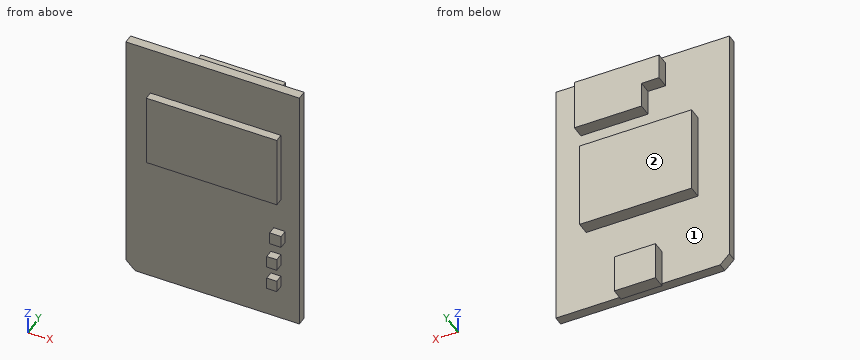
from build123d import *

# Parameters (mm, degrees)
BOSS_EXTRUDE1_DEPTH = 1.6
SKETCH3_W           = 19.355079094
SKETCH3_H           = 15.609116434
BOSS_EXTRUDE2_DEPTH = 2.2
SKETCH4_W           = 7.104895368
SKETCH4_H           = 6.377418
SKETCH4_H_2         = 0.4
BOSS_EXTRUDE4_DEPTH = 2.2
SKETCH5_W           = 22.566472962
SKETCH5_H           = 12.815854083
BOSS_EXTRUDE5_DEPTH = 1.4
SKETCH6_W           = 1.734301273
SKETCH6_H           = 2.066889472
SKETCH6_H_2         = 2.110641646
SKETCH6_W_2         = 1.994894676
SKETCH6_H_3         = 2.153908206
BOSS_EXTRUDE6_DEPTH = 1.4
SKETCH7_W           = 11.606028653
SKETCH7_H           = 9.032244077
SKETCH7_W_2         = 3.035472579
SKETCH7_H_2         = 4.516122038
BOSS_EXTRUDE7_DEPTH = 2.2


with BuildPart() as part:
    # Sketch2 → Boss-Extrude1 (new body)
    with BuildSketch(Plane(origin=(0, 0, 0), x_dir=(1, 0, 0), z_dir=(0, 1, 0))):
        Polygon((1.6, 45), (0, 43.4), (0, 0), (30, 0), (30, 45), align=None)
    extrude(amount=BOSS_EXTRUDE1_DEPTH)

    # Sketch3 → Boss-Extrude2 (add)
    with BuildSketch(Plane(origin=(0, 1.6, 0), x_dir=(1, 0, 0), z_dir=(0, 1, 0))):
        with Locations((15.091884819, 22.082133677)):
            Rectangle(SKETCH3_W, SKETCH3_H)
    extrude(amount=BOSS_EXTRUDE2_DEPTH)

    # Sketch4 → Boss-Extrude4 (add)
    with BuildSketch(Plane(origin=(0, 1.6, 0), x_dir=(1, 0, 0), z_dir=(0, 1, 0))):
        with Locations((15.215017688, 41.811291)):
            Rectangle(SKETCH4_W, SKETCH4_H)
        with Locations((15.215017688, 45.2)):
            Rectangle(SKETCH4_W, SKETCH4_H_2)
    extrude(amount=BOSS_EXTRUDE4_DEPTH)

    # Sketch5 → Boss-Extrude5 (add)
    with BuildSketch(Plane(origin=(0, 0, 0), x_dir=(-1, 0, 0), z_dir=(0, -1, 0))):
        with Locations((-15.528488828, 15.010487551)):
            Rectangle(SKETCH5_W, SKETCH5_H)
    extrude(amount=BOSS_EXTRUDE5_DEPTH)

    # Sketch6 → Boss-Extrude6 (add)
    with BuildSketch(Plane(origin=(0, 0, 0), x_dir=(-1, 0, 0), z_dir=(0, -1, 0))):
        with Locations((-25.936328658, 37.693998436)):
            Rectangle(SKETCH6_W, SKETCH6_H)
        with Locations((-25.936328658, 33.41406102)):
            Rectangle(SKETCH6_W, SKETCH6_H_2)
        with Locations((-26.557976159, 28.546467775)):
            Rectangle(SKETCH6_W_2, SKETCH6_H_3)
    extrude(amount=BOSS_EXTRUDE6_DEPTH)

    # Sketch7 → Boss-Extrude7 (add)
    with BuildSketch(Plane(origin=(0, 1.6, 0), x_dir=(1, 0, 0), z_dir=(0, 1, 0))):
        with Locations((19.872075949, 5.78373458)):
            Rectangle(SKETCH7_W, SKETCH7_H)
        with Locations((12.551325333, 3.52567356)):
            Rectangle(SKETCH7_W_2, SKETCH7_H_2)
    extrude(amount=BOSS_EXTRUDE7_DEPTH)


solid = part.part
Geometry check sheet. Reference: the model listing, model coordinates, mm. Face numbers are marked on the shaded views. Give positions to 0.01 mm unless a question says otherwise; leave off trailing zeros. Loops run counter-clockwise (first coordinate to the right, second up) from the corner with the lowest first, then second, coordinate; pieces in that order, holes last. Notation, with made-up numbers: (3, -40) -> (14, -40) arc R13 cw to (14, -21) -> close; hole circle Ø8 at (19.25, -32.5). An arc over 180 degrees is marked (long way). Answer in a Markdown table with one row per item. Add a question column.
1) Cross-section at B-B on x = 9.5. Record the boundary of the cut face in (y, z).
2) Cross-section at D-D on z = -23. Record the boundary of the cut face in (x, y).
3) Draft check along Z on the marked faces 1 and 2. Enter one of: pulls with the +Z half, pulls with the -Z half, needs draft (parallel to the pull), parting line crosses it, or undercut.
4) Material ranges on probe 1 along Z at (x, y) = (13.5, 2.4); probe 2 along Z at (x, y) = (15, 2.65); probe 3 along Y at (x, z) = (6.25, -14), recorded low to high. Write a range as from..to.
5) Gauge pin test, flat ends, axial feed: P1, Ø0.5, axis at x = 18, y = 0.5, coming from the -Z side; P2, Ø1.1, axis at x = 12, y = 3, coming from the +Z side; P3, Ø0.7, axis at y = 2.5, z = -2.5, coming from the -X side. Record the tip position at first contact, or that the pin passes through.
6) Cross-section at A-A on z = -28. Record the boundary of the cut face in (x, y).
7) Cross-section at C-C on x = 24. Record the boundary of the cut face in (y, z), and give its area (3 significant figures).
Outcome:
| question | item | result |
|---|---|---|
| 1 | outline | (-1.4, -21.42) -> (0, -21.42) -> (0, -45) -> (1.6, -45) -> (1.6, -29.89) -> (3.8, -29.89) -> (3.8, -14.28) -> (1.6, -14.28) -> (1.6, 0) -> (0, 0) -> (0, -8.6) -> (-1.4, -8.6) -> close |
| 2 | outline | (0, 0) -> (30, 0) -> (30, 1.6) -> (24.77, 1.6) -> (24.77, 3.8) -> (5.41, 3.8) -> (5.41, 1.6) -> (0, 1.6) -> close |
| 3 | face 1 | undercut |
| 3 | face 2 | needs draft |
| 4 | probe 1 | z = -45.4..-38.62, -29.89..-14.28, -5.78..-1.27 |
| 4 | probe 2 | z = -45.4..-38.62, -29.89..-14.28, -10.3..-1.27 |
| 4 | probe 3 | y = -1.4..1.6 |
| 5 | P1 | stops at z = -45 |
| 5 | P2 | stops at z = -1.27 |
| 5 | P3 | stops at x = 11.03 |
| 6 | outline | (0, 0) -> (25.56, 0) -> (25.56, -1.4) -> (27.56, -1.4) -> (27.56, 0) -> (30, 0) -> (30, 1.6) -> (24.77, 1.6) -> (24.77, 3.8) -> (5.41, 3.8) -> (5.41, 1.6) -> (0, 1.6) -> close |
| 7 | outline | (-1.4, -21.42) -> (0, -21.42) -> (0, -45) -> (1.6, -45) -> (1.6, -29.89) -> (3.8, -29.89) -> (3.8, -14.28) -> (1.6, -14.28) -> (1.6, -10.3) -> (3.8, -10.3) -> (3.8, -1.27) -> (1.6, -1.27) -> (1.6, 0) -> (0, 0) -> (0, -8.6) -> (-1.4, -8.6) -> close |
| 7 | area | 144 mm^2 |
